```python
from build123d import *

# Parameters (mm, degrees)
SKETCH1_R           = 2.54
BOSS_EXTRUDE1_DEPTH = 6.35


with BuildPart() as part:
    # Sketch1 → Boss-Extrude1 (new body)
    with BuildSketch(Plane(origin=(-21.577168497, 0, 0), x_dir=(0, 0, -1), z_dir=(1, 0, 0))):
        with BuildLine():
            Line((-122.387241806, 61.361669294), (-164.013892996, 25.356612642))
            ThreePointArc((-164.013892996, 25.356612642), (-171.951392996, 17.419112642), (-164.013892996, 9.481612642))
            Line((-164.013892996, 9.481612642), (-122.387241806, 3.703044496))
            Line((-122.387241806, 3.703044496), (-122.387241806, 11.169831477))
            Line((-122.387241806, 11.169831477), (-156.229469136, 15.867774051))
            ThreePointArc((-156.229469136, 15.867774051), (-156.245156978, 19.047193392), (-157.50733564, 21.965387779))
            Line((-157.50733564, 21.965387779), (-122.387241806, 48.668462371))
            Line((-122.387241806, 48.668462371), (-122.387241806, 61.361669294))
        make_face()
        with Locations(Location((-164.013892996, 17.419112642, 0), (0, 0, 90))):
            Circle(SKETCH1_R, mode=Mode.SUBTRACT)
    extrude(amount=-BOSS_EXTRUDE1_DEPTH)


solid = part.part
```
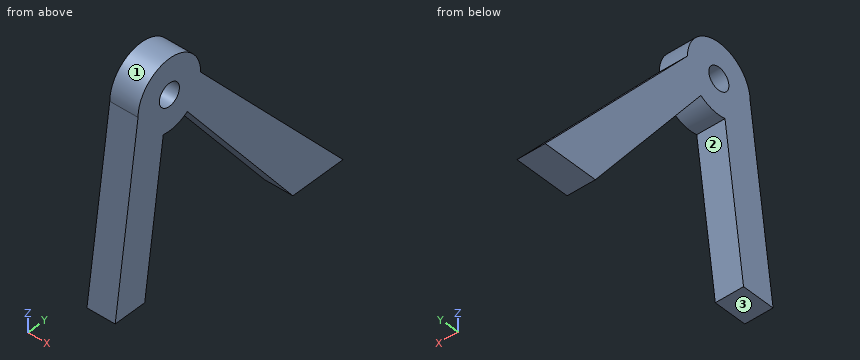
Build history of the part. All positions in model axes, mm. Face numbers are marked on the shaded views. Round coordinates to 2 decimals unless told otherwise and drop trailing zeros. Loops run counter-clockwise (first coordinate to the right, second up) from the corner with the lowest first, then second, coordinate; pieces in that order, holes last. Notation, with made-up numbers: M 58,-2.5 L 68,-2.5 A22 ccw 68,23.5 Z; hole C 15.25,63.5 d1. An arc over 180 degrees is marked long. Answer as CSV lines item,"result".
1. Flat gauge pin, fed straight in: P1, Ø1, axis at x = -27, y = 10.5, coming from the +Z side. Where does the tip first touch, or does it go through?
Resolved:
P1,"stops at z = 168.68"
2. Cut at C-C on y = 32.5. Write the cut outline in (x, z).
Resolved:
outline,"M -27.93,143.65 L -21.58,143.65 L -21.58,155.76 L -27.93,155.76 Z"
3. Two-plate mould, pull along Y, no slides. Class the marked faces 1, 2 and 3: released by +Y, released by -Y, zero draft, split by the parting line, or undercut.
Resolved:
face 1,"split by the parting line"
face 2,"undercut"
face 3,"zero draft"
4. Cut at D-D on z = 136.5. Write the cut outline in (x, y).
Resolved:
outline,"M -27.93,5.66 L -21.58,5.66 L -21.58,13.13 L -27.93,13.13 Z; M -27.93,37.94 L -21.58,37.94 L -21.58,49.15 L -27.93,49.15 Z"
5. Cut at A-A on x = -22.5. Write the cut outline in (y, z) (1 decimal).
Resolved:
outline,"M 3.7,122.4 L 11.2,122.4 L 15.9,156.2 A7.9 ccw 22,157.5 L 48.7,122.4 L 61.4,122.4 L 25.4,164 A7.9 ccw 9.5,164 Z; hole C 17.4,164 d5.1"
6. Wall check: probe 1 along Y at (x, z) = (-21.75, 138); probe 2 along Y at (x, z) = (-26.75, 150); probe 3 along Z at (x, y) = (-24, 19.5). Give the ranges that are in metal, low to high. Write a range as [from, to].
Resolved:
probe 1,"y = [5.87, 13.34], [36.8, 47.86]"
probe 2,"y = [7.54, 15], [27.67, 37.48]"
probe 3,"z = [156.35, 162.56], [165.47, 171.67]"
7. Cut at B-B on z = 130. Write the cut outline in (x, y).
Resolved:
outline,"M -27.93,4.76 L -21.58,4.76 L -21.58,12.23 L -27.93,12.23 Z; M -27.93,42.88 L -21.58,42.88 L -21.58,54.78 L -27.93,54.78 Z"
